Design review of the part built by this model. Coordinates are the model's own, in mm. A direction names the side the tool comes from. Coordinates: 2 decimals unless noted, no trailing zeros. Order: outer loops, then holes, each group sorted by start corner. A loop starts at its lowest first (then second) coordinate and runs counter-clockwise, first axis right, second up.
from build123d import *

# Parameters (mm, degrees)
BOSS_EXTRUDE1_DEPTH     = 30
BOSS_EXTRUDE2_START     = -30
BOSS_EXTRUDE2_DEPTH     = 30
CUT_EXTRUDE1_DEPTH      = 93.655275079
CUT_EXTRUDE1_DEPTH_BACK = 93.655275079
SKETCH2_R               = 2
CUT_EXTRUDE3_START      = -1
SKETCH2_3_R             = 3
CUT_EXTRUDE3_DEPTH      = 10
CUT_EXTRUDE2_DEPTH      = 93.655275079
FILLET1_R               = 4
FILLET2_R               = 3


with BuildPart() as part:
    # Sketch1 → Boss-Extrude1 (new body)
    with BuildSketch(Plane.XY):
        with BuildLine():
            Line((0, 0), (18, 0))
            Line((18, 0), (18, 32))
            Line((18, 32), (51, 32))
            ThreePointArc((51, 32), (58.071067812, 29.071067812), (61, 22))
            Line((61, 22), (61, 0))
            Line((61, 0), (79, 0))
            Line((79, 0), (79, 4))
            Line((79, 4), (65, 4))
            Line((65, 4), (65, 26))
            ThreePointArc((65, 26), (62.071067812, 33.071067812), (55, 36))
            Line((55, 36), (14, 36))
            Line((14, 36), (14, 4))
            Line((14, 4), (0, 4))
            Line((0, 4), (0, 0))
        make_face()
    extrude(amount=BOSS_EXTRUDE1_DEPTH)

    # Sketch4 → Boss-Extrude2 (add)
    with BuildSketch(Plane.XY.offset(30).offset(BOSS_EXTRUDE2_START)):
        with BuildLine():
            Line((79, 6), (67, 6))
            Line((67, 6), (67, 26))
            ThreePointArc((67, 26), (63.485281374, 34.485281374), (55, 38))
            Line((55, 38), (12, 38))
            Line((12, 38), (12, 6))
            Line((12, 6), (0, 6))
            Line((0, 6), (0, 4))
            Line((0, 4), (14, 4))
            Line((14, 4), (14, 36))
            Line((14, 36), (55, 36))
            ThreePointArc((55, 36), (62.071067812, 33.071067812), (65, 26))
            Line((65, 26), (65, 4))
            Line((65, 4), (79, 4))
            Line((79, 4), (79, 6))
        make_face()
    extrude(amount=BOSS_EXTRUDE2_DEPTH)

    # Sketch2 (on Top Plane) → Cut-Extrude1 (cut, two sides: drawn at the far end of the back side and taken through both)
    with BuildSketch(Plane(origin=(0, 0, 0), x_dir=(1, 0, 0), z_dir=(0, 1, 0)).offset(-CUT_EXTRUDE1_DEPTH_BACK)):
        with Locations(Location((6, -7, 0), (0, 0, 270))):
            Circle(SKETCH2_R)
        with Locations(Location((6, -23, 0), (0, 0, 270))):
            Circle(SKETCH2_R)
        with Locations(Location((73, -7, 0), (0, 0, 270))):
            Circle(SKETCH2_R)
        with Locations(Location((73, -23, 0), (0, 0, 270))):
            Circle(SKETCH2_R)
    extrude(amount=CUT_EXTRUDE1_DEPTH + CUT_EXTRUDE1_DEPTH_BACK, mode=Mode.SUBTRACT)

    # Sketch2<3> → Cut-Extrude3 (cut)
    with BuildSketch(Plane(origin=(0, 4, 0), x_dir=(1, 0, 0), z_dir=(0, 1, 0)).offset(CUT_EXTRUDE3_START)):
        with Locations(Location((6, -7, 0), (0, 0, 270))):
            Circle(SKETCH2_3_R)
        with Locations(Location((6, -23, 0), (0, 0, 270))):
            Circle(SKETCH2_3_R)
        with Locations(Location((73, -7, 0), (0, 0, 270))):
            Circle(SKETCH2_3_R)
        with Locations(Location((73, -23, 0), (0, 0, 270))):
            Circle(SKETCH2_3_R)
    extrude(amount=CUT_EXTRUDE3_DEPTH, mode=Mode.SUBTRACT)

    # Sketch3 → Cut-Extrude2 (cut, through all)
    with BuildSketch(Plane.XY.offset(30)):
        with BuildLine():
            ThreePointArc((55.768474142, 30.789860884), (59.593158366, 27.114452981), (61, 22))
            Line((61, 22), (61, 26.007623502))
            ThreePointArc((61, 26.007623502), (58.735019606, 28.782480547), (55.768474142, 30.789860884))
        make_face()
    extrude(amount=-CUT_EXTRUDE2_DEPTH, mode=Mode.SUBTRACT)

    # Fillet1
    fillet1_edges = [part.edges().sort_by_distance(p)[0] for p in [
        (12, 38, 15),
    ]]
    fillet(fillet1_edges, radius=FILLET1_R)

    # Fillet2
    fillet2_edges = [part.edges().sort_by_distance(p)[0] for p in [
        (12, 6, 15),
        (67, 6, 15),
    ]]
    fillet(fillet2_edges, radius=FILLET2_R - 0.0001)  # a hair under: the kernel refuses the full size


solid = part.part
1. Mouldability with a two-part tool opening along X and no side actions: class faces 5 (the cylindrical face through (13.141, 36.797, 15.21)), 6 (the flat face through (42, 33, 0)), 7 (the cylindrical face through (4.2, 4.5, 20.6)) as pulls with the +X half, pulls with the -X half, needs draft (parallel to the pull), parting line crosses it, or undercut.
2. Add section C-C (x = 6). Give the boundary of the cut face in (y, z), and give its area (3 significant figures).
3. To check wall thickness, follow line 1 (Z direction, x = 6, y = 0.65); line 2 (X direction, y = 4.45, z = 23); line 3 (Z direction, x = 73, y = 5.3). State the ranges of each line that lie inside material, in increasing order.
4. Add section D-D (y = 12). Give the boundary of the cut face in (x, z).
5. Add section B-B (z = 7). State how many separate pieces and enclosed holes the cut face has, and give its area (3 significant figures).
6. For faces 1 (the cylindrical face through (58.77, 28.75, 15.21)), 2 (the flat face through (71, 3, 24)), 3 (the flat face through (5, 6, 15)), 4 (the cylindrical face through (67.86, 6.9, 15.21)), list the 3-axis set-ups (+Z, -Z, +X, -X, +Y, -Y) from which the entire face can be reached by the end or side of a thin tool; tool diameter is ignored.
7. Insertion check: pin 1 (8.5 mm diameter, centred on y = 17, z = 16, fed in from +X); pin 2 (5 mm diameter, centred on x = 73, z = 23, fed in from +Y); pin 3 (2 mm diameter, centred on y = 10.5, z = 21.5, fed in from -X). Each pin has a flat end and moves straight along its axis. Give the tip position at first contact, or say it passes through.
8. Add section A-A (y = 5). Give the boundary of the cut face in (x, z), and give its area (3 significant figures).
Solution:
1. face 5: pulls with the -X half
1. face 6: needs draft
1. face 7: undercut
2. outline: (0, 0) - (6, 0) - (6, 4) - (3, 4) - (3, 5) - (0, 5) - close; (0, 9) - (3, 9) - (3, 10) - (6, 10) - (6, 20) - (3, 20) - (3, 21) - (0, 21) - close; (0, 25) - (3, 25) - (3, 26) - (6, 26) - (6, 30) - (0, 30) - close
2. area: 120 mm2
3. line 1: z = 0 to 5, 9 to 21, 25 to 30
3. line 2: x = 0 to 3, 9 to 18, 61 to 70, 76 to 79
3. line 3: z = 0 to 4, 10 to 20, 26 to 30
4. outline: (12, 0) - (18, 0) - (18, 30) - (12, 30) - close; (61, 0) - (67, 0) - (67, 30) - (61, 30) - close
5. separate pieces: 3
5. enclosed holes: 0
5. area: 786 mm2
6. face 1: +Z, -Z, -Y
6. face 2: +Y
6. face 3: +Z, -Z, -X, +Y
6. face 4: +Z, -Z, +X, +Y
7. pin 1: stops at x = 67
7. pin 2: stops at y = 3
7. pin 3: stops at x = 12
8. outline: (0, 0) - (18, 0) - (18, 30) - (0, 30) - close; (61, 0) - (79, 0) - (79, 30) - (61, 30) - close; hole circle Ø6 at (6, 7); hole circle Ø6 at (6, 23); hole circle Ø6 at (73, 7); hole circle Ø6 at (73, 23)
8. area: 967 mm2
